The listing builds one solid part. Answer for the finished solid, in the listing's coordinates (mm). Coordinates: 2 decimals unless noted, no trailing zeros. Use one line per item in the form item = value. Start each with the question number.
```python
from build123d import *

# Parameters (mm, degrees)
BOSS_EXTRUDE1_DEPTH = 750


with BuildPart() as part:
    # Sketch1 → Boss-Extrude1 (new body)
    with BuildSketch(Plane(origin=(-10, 0, 0), x_dir=(0, 0, -1), z_dir=(1, 0, 0))):
        with BuildLine():
            Line((-14, 20.148439), (-14, 18.35158))
            ThreePointArc((-14, 18.35158), (-13.885407957, 18.031881418), (-13.592386868, 17.860192277))
            ThreePointArc((-13.592386868, 17.860192277), (-12.229021504, 17.099202354), (-11.602627372, 15.66899217))
            ThreePointArc((-11.602627372, 15.66899217), (-11.559004129, 15.501191683), (-11.458152391, 15.360163609))
            Line((-11.458152391, 15.360163609), (-11.005017, 14.906991))
            ThreePointArc((-11.005017, 14.906991), (-10.852063473, 14.680418582), (-10.800003, 14.412054))
            Line((-10.800003, 14.412054), (-10.800003, 10.490777069))
            ThreePointArc((-10.800003, 10.490777069), (-10.853443426, 10.222114259), (-11.005628687, 9.994352913))
            Line((-11.005628687, 9.994352913), (-13.795574427, 7.204407575))
            ThreePointArc((-13.795574427, 7.204407575), (-13.946871354, 6.977976046), (-14, 6.710881784))
            Line((-14, 6.710881784), (-14, 1.5))
            Line((-14, 1.5), (-12.5, 0))
            Line((-12.5, 0), (12.5, 0))
            Line((12.5, 0), (14, 1.5))
            Line((14, 1.5), (14, 6.710881784))
            ThreePointArc((14, 6.710881784), (13.946871354, 6.977976046), (13.795574427, 7.204407575))
            Line((13.795574427, 7.204407575), (11.005628687, 9.994352913))
            ThreePointArc((11.005628687, 9.994352913), (10.853443426, 10.222114259), (10.800003, 10.490777069))
            Line((10.800003, 10.490777069), (10.800003, 14.412054))
            ThreePointArc((10.800003, 14.412054), (10.852063473, 14.680418582), (11.005017, 14.906991))
            Line((11.005017, 14.906991), (11.458152391, 15.360163609))
            ThreePointArc((11.458152391, 15.360163609), (11.559004129, 15.501191683), (11.602627372, 15.66899217))
            ThreePointArc((11.602627372, 15.66899217), (12.229021504, 17.099202354), (13.592386868, 17.860192277))
            ThreePointArc((13.592386868, 17.860192277), (13.885407957, 18.031881418), (14, 18.35158))
            Line((14, 18.35158), (14, 20.148439))
            ThreePointArc((14, 20.148439), (13.886532321, 20.469052961), (13.5924176, 20.639829881))
            ThreePointArc((13.5924176, 20.639829881), (12.312672018, 21.314596081), (11.635789981, 22.593223817))
            ThreePointArc((11.635789981, 22.593223817), (11.466717508, 22.887148006), (11.146965482, 23))
            Line((11.146965482, 23), (-11.146965482, 23))
            ThreePointArc((-11.146965482, 23), (-11.466717508, 22.887148006), (-11.635789981, 22.593223817))
            ThreePointArc((-11.635789981, 22.593223817), (-12.312672018, 21.314596081), (-13.5924176, 20.639829881))
            ThreePointArc((-13.5924176, 20.639829881), (-13.886532321, 20.469052961), (-14, 20.148439))
        make_face()
    extrude(amount=BOSS_EXTRUDE1_DEPTH)

    # Sketch2 → Cut-Revolve1 (revolve, cut)
    with BuildSketch(Plane.XY, mode=Mode.PRIVATE) as cut_revolve1_sk:
        Polygon((0, 23), (7, 23), (7, 11), (4.5, 11), (4.5, 0), (0, 0), align=None)
    revolve(cut_revolve1_sk.sketch.rotate(Axis((0, 0, 0), (0, 1, 0)), 270), axis=Axis((0, 0, 0), (0, 1, 0)), mode=Mode.SUBTRACT)

    # Sketch3 → Cut-Revolve2 (revolve, cut)
    with BuildSketch(Plane.XY, mode=Mode.PRIVATE) as cut_revolve2_sk:
        Polygon((80, 23), (87, 23), (87, 11), (84.5, 11), (84.5, 0), (80, 0), align=None)
    revolve(cut_revolve2_sk.sketch.rotate(Axis((80, 0, 0), (0, 1, 0)), 270), axis=Axis((80, 0, 0), (0, 1, 0)), mode=Mode.SUBTRACT)

    # Sketch4 → Cut-Revolve3 (revolve, cut)
    with BuildSketch(Plane.XY, mode=Mode.PRIVATE) as cut_revolve3_sk:
        Polygon((160, 23), (167, 23), (167, 11), (164.5, 11), (164.5, 0), (160, 0), align=None)
    revolve(cut_revolve3_sk.sketch.rotate(Axis((160, 0, 0), (0, 1, 0)), 270), axis=Axis((160, 0, 0), (0, 1, 0)), mode=Mode.SUBTRACT)

    # Sketch5 → Cut-Revolve4 (revolve, cut)
    with BuildSketch(Plane.XY, mode=Mode.PRIVATE) as cut_revolve4_sk:
        Polygon((240, 23), (247, 23), (247, 11), (244.5, 11), (244.5, 0), (240, 0), align=None)
    revolve(cut_revolve4_sk.sketch.rotate(Axis((240, 0, 0), (0, 1, 0)), 270), axis=Axis((240, 0, 0), (0, 1, 0)), mode=Mode.SUBTRACT)

    # Sketch6 → Cut-Revolve5 (revolve, cut)
    with BuildSketch(Plane.XY, mode=Mode.PRIVATE) as cut_revolve5_sk:
        Polygon((320, 23), (327, 23), (327, 11), (324.5, 11), (324.5, 0), (320, 0), align=None)
    revolve(cut_revolve5_sk.sketch.rotate(Axis((320, 0, 0), (0, 1, 0)), 270), axis=Axis((320, 0, 0), (0, 1, 0)), mode=Mode.SUBTRACT)

    # Sketch7 → Cut-Revolve6 (revolve, cut)
    with BuildSketch(Plane.XY, mode=Mode.PRIVATE) as cut_revolve6_sk:
        Polygon((400, 23), (407, 23), (407, 11), (404.5, 11), (404.5, 0), (400, 0), align=None)
    revolve(cut_revolve6_sk.sketch.rotate(Axis((400, 0, 0), (0, 1, 0)), 270), axis=Axis((400, 0, 0), (0, 1, 0)), mode=Mode.SUBTRACT)

    # Sketch8 → Cut-Revolve7 (revolve, cut)
    with BuildSketch(Plane.XY, mode=Mode.PRIVATE) as cut_revolve7_sk:
        Polygon((480, 23), (487, 23), (487, 11), (484.5, 11), (484.5, 0), (480, 0), align=None)
    revolve(cut_revolve7_sk.sketch.rotate(Axis((480, 0, 0), (0, 1, 0)), 270), axis=Axis((480, 0, 0), (0, 1, 0)), mode=Mode.SUBTRACT)


solid = part.part
```
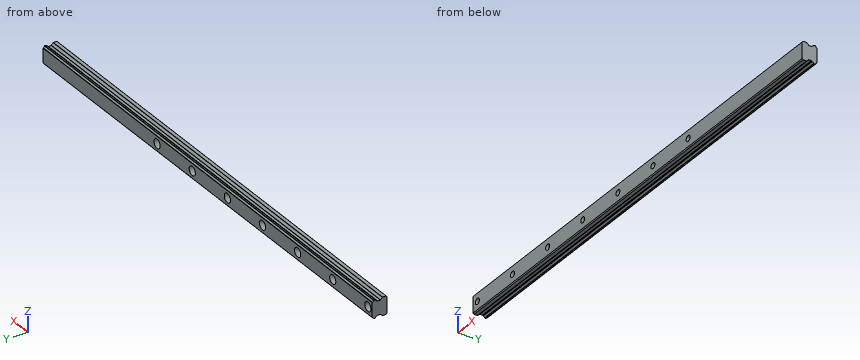
(1) A cutting plane is placed at A-A (z = 0). State how many separate pieces and enclosed holes the cut face has, then the cut area to 3 significant figures.
(2) Each of these flat-tipped pins is pushed along its axis until it touches: pin 1 Ø1.5 at (x, y) = (138.5, 9.5) entering from -Z; pin 2 Ø8.5 at (x, z) = (400, 0) entering from +Y; pin 3 Ø1.5 at (x, y) = (543.5, 9) entering from -Z; pin 4 Ø3 at (x, y) = (537.5, 12) entering from +Z. Where does it stop, or does it pass through?
(3) Find the intervals of material crossed by probe 1 along Z at (x, y) = (320, 14.25); probe 2 along Z at (x, y) = (401, 7.5); probe 3 along Y at (x, z) = (215, 12.5), in increasing order. Write a range as from..to.
Evaluation:
q1.separate_pieces = 8
q1.enclosed_holes = 0
q1.area = 15,400 mm^2
q2.pin_1 = -12.25
q2.pin_2 = through
q2.pin_3 = -12.75
q2.pin_4 = 10.8
q3.probe_1 = -10.8..-7, 7..10.8
q3.probe_2 = -13.5..-4.39, 4.39..13.5
q3.probe_3 = 0..8.5, 17.36..21.15
